from build123d import *

# Parameters (mm, degrees)
CUT_EXTRUDE3_DEPTH         = 1.4478
DRAFT1_ANGLE               = -20
RECESSI_CUT_EXTRUDE5_DEPTH = 1.4478


with BuildPart() as part:
    # Sketch1 → base-Revolve (revolve)
    with BuildSketch(Plane.XY, mode=Mode.PRIVATE) as base_revolve_sk:
        with BuildLine():
            Line((0.33207054, 2.358608179), (1.4478, 1.4224))
            Line((1.4478, 1.4224), (11.1125, 1.4224))
            Line((11.1125, 1.4224), (11.1125, 0))
            Line((11.1125, 0), (0, 0))
            Line((0, 0), (-0.7366, 0))
            ThreePointArc((-0.7366, 0), (-0.604667324, 1.151304479), (-0.215709527, 2.242917995))
            ThreePointArc((-0.215709527, 2.242917995), (0.030014098, 2.434127878), (0.33207054, 2.358608179))
        make_face()
    revolve(base_revolve_sk.sketch.rotate(Axis((0, 0, 0), (1, 0, 0)), 90), axis=Axis((0, 0, 0), (1, 0, 0)))

    # Sketch4 → Cut-Extrude3 (cut)
    with BuildSketch(Plane(origin=(-0.7366, 0, 0), x_dir=(0, 0, -1), z_dir=(1, 0, 0))):
        Polygon((0.2413, 1.4986), (-0.2413, 1.4986), (-0.2413, 0.2413), (-1.4986, 0.2413), (-1.4986, -0.2413), (-0.2413, -0.2413), (-0.2413, -1.4986), (0.2413, -1.4986), (0.2413, -0.2413), (1.4986, -0.2413), (1.4986, 0.2413), (0.2413, 0.2413), align=None)
    extrude(amount=CUT_EXTRUDE3_DEPTH, mode=Mode.SUBTRACT)

    # Draft1
    draft1_faces = [part.faces().sort_by_distance(p)[0] for p in [
        (0.101115896, 0, -1.4986),
        (0.101115896, -1.4986, 0),
        (0.101115896, 0, 1.4986),
        (0.101115896, 1.4986, 0),
    ]]
    draft(draft1_faces, Plane(origin=(-0.7366, 0, 0), x_dir=(0, 0, 1), z_dir=(1, 0, 0)), DRAFT1_ANGLE)

    # Sketch5 → recessI_Cut-Extrude5 (cut)
    with BuildSketch(Plane.ZY.offset(0.7366)):
        Polygon((0.2413, 0.54102), (0.54102, 0.2413), (0.2413, 0.2413), align=None)
        Polygon((-0.2413, 0.2413), (-0.54102, 0.2413), (-0.2413, 0.54102), align=None)
        Polygon((-0.2413, -0.54102), (-0.54102, -0.2413), (-0.2413, -0.2413), align=None)
        Polygon((0.2413, -0.2413), (0.54102, -0.2413), (0.2413, -0.54102), align=None)
    extrude(amount=-RECESSI_CUT_EXTRUDE5_DEPTH, mode=Mode.SUBTRACT)

    # Sketch8 → point_Cut-Revolve1 (revolve, cut)
    with BuildSketch(Plane.XY, mode=Mode.PRIVATE) as point_cut_revolve1_sk:
        Polygon((11.1125, 0), (11.6205, 0), (11.6205, 1.9304), (10.386597507, 1.9304), (10.386597507, 1.4224), (11.1125, 1.0033), align=None)
    revolve(point_cut_revolve1_sk.sketch.rotate(Axis((0, 0, 0), (1, 0, 0)), 90), axis=Axis((0, 0, 0), (1, 0, 0)), mode=Mode.SUBTRACT)


solid = part.part
Read the model definition and answer for the solid it produces. Units are mm, in the model's axes. Give positions to 0.01 mm unless a question says otherwise; leave off trailing zeros. Write each loop counter-clockwise with the first axis right and the second up, starting at its lowest first coordinate (ties: lowest second). Pieces come first, ordered by that corner, then holes. Notation, with made-up numbers: (-33, 45.25) - (8, 45.25) arc R18 cw to (8, 77.25) - close; hole circle Ø2 at (51.25, 37). An arc over 180 degrees is marked (long way). Return JSON: item names as keys, results as strings.
Q1. A cutting plane is placed at A-A, the plane y = 0. Determine the outline of the cut face in (x, z), and give its area (3 significant figures).
Reply:
{"outline": "(-0.53, -1.42) arc R5.09 ccw to (-0.22, -2.24) arc R0.36 ccw to (0.33, -2.36) - (1.45, -1.42) - (10.39, -1.42) - (11.11, -1) - (11.11, 1) - (10.39, 1.42) - (1.45, 1.42) - (0.33, 2.36) arc R0.36 ccw to (-0.22, 2.24) arc R5.09 ccw to (-0.53, 1.42) - (0.71, 0.97) - (0.71, -0.97) - close", "area": "32.2 mm²"}
Q2. Consider line 1 along X through (y, z) = (-0.1, 0.2); line 2 along Y through (x, z) = (9.5, -0.1); line 3 along Y through (x, z) = (1.75, 1.2). Determine where each line is inside the solid, lowest interval first. Write a range as [from, to].
Reply:
{"line 1": "[0.71, 11.11]", "line 2": "[-1.42, 1.42]", "line 3": "[-0.76, 0.76]"}
Q3. Given P1, Ø1, axis at x = 7, z = 1.5, coming from the +Y side; P2, Ø1, axis at x = 0, z = 1, coming from the -Y side; P3, Ø2, axis at x = 4.5, z = 2, coming from the -Y side; P4, Ø0.6, axis at y = 0.5, z = 0, coming from the -X side, each flat-ended and moving along its own axis, determine where each tip first touches the part or whether it passes through.
Reply:
{"P1": "y = 1.01", "P2": "y = -2.39", "P3": "y = -1.01", "P4": "x = -0.7"}
Q4. For a pull along Y with two mould halves and no side action, classify faces 1 (the face through (0, 0.241, 1)), 2 (the face through (11.112, 0, 0)), 3 (the face through (5.98, 1.26, 0.66)) as released by +Y, released by -Y, zero draft, split by the parting line, or undercut.
Reply:
{"face 1": "undercut", "face 2": "zero draft", "face 3": "split by the parting line"}
Q5. A cutting plane is placed at C-C, the plane x = 2. Determine the outline of the cut face in (y, z).
Reply:
{"outline": "circle Ø2.84 at (0, 0)"}
